The figure shows three views and two pictorial views of one solid part (mm, origin at its lowest corner). Answer the questions. A direction names the side the tool comes from. Give positions to 0.01 mm unless a question says otherwise; leave off trailing zeros. Write each loop counter-clockwise with the first axis right and the second up, starting at its lowest first coordinate (ties: lowest second). Pieces come first, ordered by that corner, then holes. Notation, with made-up numbers: (-19.5, 80.25) -> (-11.5, 80.25) arc R23 ccw to (-11.5, 88.25) -> close; hole circle Ø1 at (8.5, 37.5). An arc over 180 degrees is marked (long way). Write each question's results on one line, items separated by ' | '. Start each with the question number.
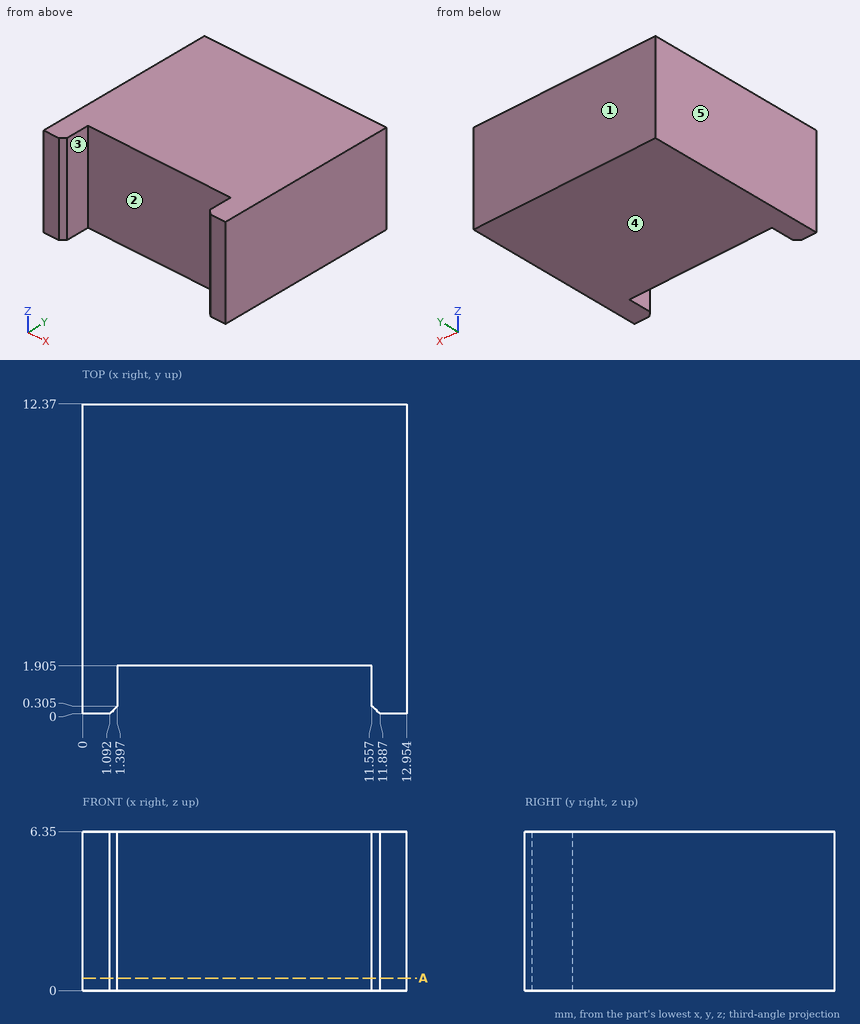
1. A tool of negligible diameter and unlimited length cuts with its end or side. For the marked faces 1 and 2, from which of +Z, -Z, +X, -X, +Y, -Y can it reach the whole face along a straight path? Write none if from no direction.
2. The mould has two halves that part along X. Classify the marked faces 3, 4 and 5: pulls with the +X half, pulls with the -X half, needs draft (parallel to the pull), parting line crosses it, or undercut.
3. This flat-tipped pin is pushed along its axis until it touches: pin 1 Ø1.9 at (x, z) = (7.5, 3) entering from -Y (3 decimals). Where does it stop, or does it pass through?
4. Consider probe 1 along X at (y, z) = (0.5, 1); probe 2 along Y at (x, z) = (5.25, 5.5) (1 decimal); probe 3 along Y at (x, z) = (1.25, 1). Determine where each line is inside the solid, lowest interval first. Write a range as [from, to].
5. Section A-A (z = 0.5) is taken. Write down the section's boundary in (x, y) (1 decimal), then the cut area to 3 significant figures.
Results:
1) face 1: +Z, -Z, +X, -X, +Y | face 2: +Z, -Z, -Y
2) face 3: undercut | face 4: needs draft | face 5: pulls with the -X half
3) pin 1: stops at y = 1.905
4) probe 1: x = [0, 1.4], [11.56, 12.95] | probe 2: y = [1.9, 12.4] | probe 3: y = [0.16, 12.37]
5) outline: (0, 0) -> (1.1, 0) -> (1.4, 0.3) -> (1.4, 1.9) -> (11.6, 1.9) -> (11.6, 0.3) -> (11.9, 0) -> (13, 0) -> (13, 12.4) -> (0, 12.4) -> close | area: 141 mm²
